Model file for the job. Use its own axes, mm. A direction names the side the tool comes from. Coordinates: 2 decimals unless noted, no trailing zeros. Write each loop counter-clockwise with the first axis right and the second up, starting at its lowest first coordinate (ties: lowest second). Pieces come first, ordered by that corner, then holes. Notation, with made-up numbers: M 39.25,41.25 L 83.25,41.25 A6 cw 83.25,45.25 Z; hole C 27.25,71.5 d5. An arc over 180 degrees is marked long. Put each result on its own line as item: value. Start each with the question number.
Q1. Cut at A-A (x = 52). Write the cut outline in (y, z).
Q2. Pull direction Z, two halves, no side cores. Call faces 6 (the flat face through (1, 1, -24.599)), 7 (the flat face through (63, 1, -3)), 8 (the flat face through (37.779, 1, -2)): pulls with the +Z half, pulls with the -Z half, needs draft (parallel to the pull), parting line crosses it, or undercut.
Q3. Drill centre lines: line 1 along Z through (x, y) = (21, 0.85); line 2 along X through (y, z) = (1.35, -3.5). Where is each one in solid material? Low to high.
Q4. Cut at C-C (y = 1.1). Give the number of separate pieces and of enclosed holes in the cut face, then the cut area to 3 significant figures.
Q5. Cut at B-B (z = -21.5). Write the cut outline in (x, y), then the cut area to 3 significant figures.
Q6. Which spindle directions (+Z, -Z, +X, -X, +Y, -Y) get a long thin tool onto all of the face, cutting with end or side? Do faces 1 (the flat face through (30.223, 1, -1)), 2 (the flat face through (66, 1, -8.199)), 3 (the flat face through (5, 1, -3)), 4 (the flat face through (2, 1, -16.4)), 5 (the flat face through (34, 1, -37.999)). Say none if no direction does.
Q7. Drop flat-ended pins along their axis: pin 1 (1.7 mm diameter, centred on x = 61.5, z = -34.5, fed in from +Y); pin 2 (1.5 mm diameter, centred on y = 1.5, z = -1.5, fed in from -X); pin 3 (1.2 mm diameter, centred on x = 6.5, z = -6.5, fed in from -Y); pin 4 (1.5 mm diameter, centred on y = 1.5, z = -35.5, fed in from -X). Give the stop position or say it passes through.
```python
from build123d import *

# Parameters (mm, degrees)
AUFSATZ_LINEAR_AUSTRAGEN1_DEPTH = 3
SCHNITT_LINEAR_AUSTRAGEN1_REACH = 5
SKIZZE2_R                       = 0.65


with BuildPart() as part:
    # Skizze1 → Aufsatz-Linear austragen1 (new body)
    with BuildSketch(Plane(origin=(0, 0, 0), x_dir=(1, 0, 0), z_dir=(0, 1, 0))):
        Polygon((2.999994, 37.999416), (2.999994, 32.800036), (0, 32.800036), (0, 24.599138), (2.999994, 24.599138), (2.999994, 16.399764), (0, 16.399764), (0, 8.19912), (2.999994, 8.19912), (2.999994, 2.999994), (7.555738, 2.999994), (7.555738, 0), (15.11173, 0), (15.11173, 2.999994), (22.667468, 2.999994), (22.667468, 0), (30.223206, 0), (30.223206, 2.999994), (37.778944, 2.999994), (37.778944, 0), (45.333412, 0), (45.333412, 2.999994), (52.88915, 2.999994), (52.88915, 0), (60.444888, 0), (60.444888, 2.999994), (65.000632, 2.999994), (65.000632, 8.19912), (68.00088, 8.19912), (68.00088, 16.399764), (65.000632, 16.399764), (65.000632, 24.599138), (68.00088, 24.599138), (68.00088, 32.800036), (65.000632, 32.800036), (65.000632, 37.999416), (60.444888, 37.999416), (60.444888, 40.99941), (52.88915, 40.99941), (52.88915, 37.999416), (45.333412, 37.999416), (45.333412, 40.99941), (37.778944, 40.99941), (37.778944, 37.999416), (30.223206, 37.999416), (30.223206, 40.99941), (22.667468, 40.99941), (22.667468, 37.999416), (15.11173, 37.999416), (15.11173, 40.99941), (7.555738, 40.99941), (7.555738, 37.999416), align=None)
    extrude(amount=AUFSATZ_LINEAR_AUSTRAGEN1_DEPTH)

    # Skizze2 → Schnitt-Linear austragen1 (cut, up to next)
    with BuildSketch(Plane(origin=(0, 3, 0), x_dir=(1, 0, 0), z_dir=(0, 1, 0)), mode=Mode.PRIVATE) as schnitt_linear_austragen1_sk1:
        with Locations((6.501075, 34.499451)):
            Circle(SKIZZE2_R)
    schnitt_linear_austragen1_tool1 = extrude(schnitt_linear_austragen1_sk1.sketch, amount=-SCHNITT_LINEAR_AUSTRAGEN1_REACH, mode=Mode.PRIVATE) & part.part
    add(schnitt_linear_austragen1_tool1.solids().sort_by_distance((6.501075, 3, -34.499451))[0], mode=Mode.SUBTRACT)
    # Skizze2 → Schnitt-Linear austragen1 (cut, up to next)
    with BuildSketch(Plane(origin=(0, 3, 0), x_dir=(1, 0, 0), z_dir=(0, 1, 0)), mode=Mode.PRIVATE) as schnitt_linear_austragen1_sk2:
        with Locations((61.501075, 34.499451)):
            Circle(SKIZZE2_R)
    schnitt_linear_austragen1_tool2 = extrude(schnitt_linear_austragen1_sk2.sketch, amount=-SCHNITT_LINEAR_AUSTRAGEN1_REACH, mode=Mode.PRIVATE) & part.part
    add(schnitt_linear_austragen1_tool2.solids().sort_by_distance((61.501075, 3, -34.499451))[0], mode=Mode.SUBTRACT)
    # Skizze2 → Schnitt-Linear austragen1 (cut, up to next)
    with BuildSketch(Plane(origin=(0, 3, 0), x_dir=(1, 0, 0), z_dir=(0, 1, 0)), mode=Mode.PRIVATE) as schnitt_linear_austragen1_sk3:
        with Locations((61.501075, 6.499451)):
            Circle(SKIZZE2_R)
    schnitt_linear_austragen1_tool3 = extrude(schnitt_linear_austragen1_sk3.sketch, amount=-SCHNITT_LINEAR_AUSTRAGEN1_REACH, mode=Mode.PRIVATE) & part.part
    add(schnitt_linear_austragen1_tool3.solids().sort_by_distance((61.501075, 3, -6.499451))[0], mode=Mode.SUBTRACT)
    # Skizze2 → Schnitt-Linear austragen1 (cut, up to next)
    with BuildSketch(Plane(origin=(0, 3, 0), x_dir=(1, 0, 0), z_dir=(0, 1, 0)), mode=Mode.PRIVATE) as schnitt_linear_austragen1_sk4:
        with Locations((6.501075, 6.499451)):
            Circle(SKIZZE2_R)
    schnitt_linear_austragen1_tool4 = extrude(schnitt_linear_austragen1_sk4.sketch, amount=-SCHNITT_LINEAR_AUSTRAGEN1_REACH, mode=Mode.PRIVATE) & part.part
    add(schnitt_linear_austragen1_tool4.solids().sort_by_distance((6.501075, 3, -6.499451))[0], mode=Mode.SUBTRACT)


solid = part.part
```
Computed values:
1. outline: M 0,-38 L 3,-38 L 3,-3 L 0,-3 Z
2. face 6: undercut
2. face 7: pulls with the +Z half
2. face 8: needs draft
3. line 1: -38 to -3
3. line 2: 3 to 65
4. separate pieces: 1
4. enclosed holes: 4
4. area: 2,440 mm2
5. outline: M 3,0 L 65,0 L 65,3 L 3,3 Z
5. area: 186 mm2
6. face 1: +Z, +Y, -Y
6. face 2: +Z, +X, +Y, -Y
6. face 3: +Z, -X, +Y, -Y
6. face 4: -X, +Y, -Y
6. face 5: -Z, +Y, -Y
7. pin 1: y = 3
7. pin 2: x = 7.56
7. pin 3: through
7. pin 4: x = 3
